CAD build for the part. Positions are in the model's coordinates, mm. A direction names the side the tool comes from. Give positions to 0.01 mm unless a question says otherwise; leave off trailing zeros. Write each loop counter-clockwise with the first axis right and the second up, starting at its lowest first coordinate (ties: lowest second). Pieces come first, ordered by that corner, then holes. Notation, with made-up numbers: (43.25, -26) - (99.25, -26) arc R29 ccw to (99.25, 7) - close; hole circle Ø3 at (8.25, -26.5). An arc over 180 degrees is marked (long way). Put each result on its own line as item: value. Start each with the question number.
1. Cut at C-C on z = 9. List the corners of the cut face in (x, y), and give its area (3 significant figures).
2. Drop flat-ended pins along their axis: pin 1 (8 mm diameter, centred on x = 21, z = -0.5, fed in from -Y); pin 2 (1 mm diameter, centred on x = 44.5, y = 4, fed in from -Z); pin 3 (8 mm diameter, centred on x = 57.5, z = 9, fed in from +Y). Give the stop position or say it passes through.
3. Mould opens along X. For faces 6 (the flat face through (68.9, -2, 9)), 7 (the flat face through (34, 5, 0)), 8 (the flat face through (1, -7, 0)) say: +X half, -X half, draft (parallel to the pull), parting line (faces both ways), or undercut.
4. Tool access for faces 1 (the flat face through (1, -2, 9)), 2 (the cylindrical face through (1.91, -5.48, -52.39)), 3 (the flat face through (21, -2, -63)), 4 (the flat face through (68.9, -2, -63)), 5 (the flat face through (11, -1, -60.9)): list every direction of +Z, -Z, +X, -X, +Y, -Y with a clear straight run to the whole face (end or side of a thin tool).
5. Cut at A-A on z = -27.2. List the corners of the cut face in (x, y).
6. Wall check: line 1 (Y direction, x = -0.45, z = -27.2); line 2 (Z direction, x = 63, y = 9.25); line 3 (Z direction, x = 12.5, y = 0.25). Give the ranges that are in metal, low to high.
7. Cut at D-D on x = 27.5. List the corners of the cut face in (y, z), and give its area (3 significant figures).
8. Cut at B-B on y = 8. List the corners of the cut face in (x, z).
from build123d import *

# Parameters (mm, degrees)
SKETCH1_W               = 77.9
SKETCH1_H               = 62.4
SKETCH1_W_2             = 69.9
SKETCH1_H_2             = 54.4
BOSS_EXTRUDE1_DEPTH     = 10
SKETCH2_W               = 77.9
SKETCH2_H               = 62.4
BOSS_EXTRUDE2_DEPTH     = 4
SKETCH7_W               = 73.9
SKETCH7_H               = 58.4
SKETCH7_W_2             = 69.9
SKETCH7_H_2             = 54.4
BOSS_EXTRUDE4_DEPTH     = 1
CUT_EXTRUDE1_REACH      = 99.979
SKETCH3_W               = 13
SKETCH3_H               = 7.25
CUT_EXTRUDE2_REACH      = 99.979
SKETCH4_W               = 10
SKETCH4_H               = 7.25
SKETCH5_R               = 1.36925
CUT_EXTRUDE4_DEPTH      = 25
SKETCH6_R               = 2.5
BOSS_EXTRUDE3_DEPTH     = 3
SKETCH9_W               = 10
SKETCH9_H               = 1
SKETCH9_W_2             = 13
CUT_EXTRUDE5_DEPTH      = 11
SKETCH11_W              = 5
SKETCH11_H              = 5
SKETCH11_R              = 1
BOSS_EXTRUDE5_DEPTH     = 2
BOSS_EXTRUDE6_START     = -2
SKETCH12_W              = 5
SKETCH12_H              = 5
SKETCH12_R              = 1
BOSS_EXTRUDE6_DEPTH     = 2
SKETCH13_W              = 20
SKETCH13_H              = 5
BOSS_EXTRUDE7_DEPTH     = 10
CUT_EXTRUDE6_DEPTH      = 10
MIRROR2_COPY_1_SKETCH_W = 20
MIRROR2_COPY_1_SKETCH_H = 5
MIRROR2_COPY_1_DEPTH    = 10
MIRROR2_COPY_2_DEPTH    = 10


with BuildPart() as part:
    # Sketch1 → Boss-Extrude1 (new body)
    with BuildSketch(Plane(origin=(0, 0, 0), x_dir=(1, 0, 0), z_dir=(0, 1, 0))):
        with Locations((34.95, 27.2)):
            Rectangle(SKETCH1_W, SKETCH1_H)
        with Locations((34.95, 27.2)):
            Rectangle(SKETCH1_W_2, SKETCH1_H_2, mode=Mode.SUBTRACT)
    extrude(amount=BOSS_EXTRUDE1_DEPTH)

    # Sketch2 → Boss-Extrude2 (add)
    with BuildSketch(Plane(origin=(0, 0, 0), x_dir=(1, 0, 0), z_dir=(0, 1, 0))):
        with Locations((34.95, 27.2)):
            Rectangle(SKETCH2_W, SKETCH2_H)
    extrude(amount=-BOSS_EXTRUDE2_DEPTH)

    # Sketch7 → Boss-Extrude4 (add)
    with BuildSketch(Plane(origin=(0, 10, 0), x_dir=(1, 0, 0), z_dir=(0, 1, 0))):
        with Locations((34.95, 27.2)):
            Rectangle(SKETCH7_W, SKETCH7_H)
        with Locations((34.95, 27.2)):
            Rectangle(SKETCH7_W_2, SKETCH7_H_2, mode=Mode.SUBTRACT)
    extrude(amount=BOSS_EXTRUDE4_DEPTH)

    # Sketch3 → Cut-Extrude1 (cut, up to next)
    with BuildSketch(Plane.ZY.offset(4), mode=Mode.PRIVATE) as cut_extrude1_sk1:
        with Locations((-38.4, 6.375)):
            Rectangle(SKETCH3_W, SKETCH3_H)
    cut_extrude1_tool1 = extrude(cut_extrude1_sk1.sketch, amount=-CUT_EXTRUDE1_REACH, mode=Mode.PRIVATE) & part.part
    add(cut_extrude1_tool1.solids().sort_by_distance((-4, 6.375, -38.4))[0], mode=Mode.SUBTRACT)

    # Sketch4 → Cut-Extrude2 (cut, up to next)
    with BuildSketch(Plane.ZY.offset(4), mode=Mode.PRIVATE) as cut_extrude2_sk1:
        with Locations((-8.5, 6.375)):
            Rectangle(SKETCH4_W, SKETCH4_H)
    cut_extrude2_tool1 = extrude(cut_extrude2_sk1.sketch, amount=-CUT_EXTRUDE2_REACH, mode=Mode.PRIVATE) & part.part
    add(cut_extrude2_tool1.solids().sort_by_distance((-4, 6.375, -8.5))[0], mode=Mode.SUBTRACT)

    # Sketch5 → Cut-Extrude4 (cut, symmetric)
    with BuildSketch(Plane(origin=(0, -4, 0), x_dir=(-1, 0, 0), z_dir=(0, -1, 0))):
        with Locations(Location((-65.94475, 7.99125, 0), (0, 0, 270))):
            Circle(SKETCH5_R)
        with Locations(Location((-15.15745, 51.15855, 0), (0, 0, 270))):
            Circle(SKETCH5_R)
        with Locations(Location((-65.94475, 35.91855, 0), (0, 0, 270))):
            Circle(SKETCH5_R)
        with Locations(Location((-14.01445, 3.24145, 0), (0, 0, 270))):
            Circle(SKETCH5_R)
    extrude(amount=CUT_EXTRUDE4_DEPTH, both=True, mode=Mode.SUBTRACT)

    # Sketch6 → Boss-Extrude3 (add)
    with BuildSketch(Plane(origin=(0, -4, 0), x_dir=(-1, 0, 0), z_dir=(0, -1, 0))):
        with Locations(Location((-0.95, -0.3, 0), (0, 0, 270))):
            Circle(SKETCH6_R)
        with Locations(Location((-0.95, 54.7, 0), (0, 0, 270))):
            Circle(SKETCH6_R)
        with Locations(Location((-68.95, 54.7, 0), (0, 0, 270))):
            Circle(SKETCH6_R)
        with Locations(Location((-68.95, -0.3, 0), (0, 0, 270))):
            Circle(SKETCH6_R)
    extrude(amount=BOSS_EXTRUDE3_DEPTH)

    # Sketch9 → Cut-Extrude5 (cut)
    with BuildSketch(Plane.ZY.offset(2)):
        with Locations((-8.5, 10.5)):
            Rectangle(SKETCH9_W, SKETCH9_H)
        with Locations((-38.4, 10.5)):
            Rectangle(SKETCH9_W_2, SKETCH9_H)
    extrude(amount=-CUT_EXTRUDE5_DEPTH, mode=Mode.SUBTRACT)

    # Sketch11 → Boss-Extrude5 (add)
    with BuildSketch(Plane(origin=(71.9, 0, 0), x_dir=(0, 0, -1), z_dir=(1, 0, 0))):
        with Locations((27.2, 12.5)):
            Rectangle(SKETCH11_W, SKETCH11_H)
        with Locations((27.2, 12.5)):
            Circle(SKETCH11_R, mode=Mode.SUBTRACT)
    extrude(amount=-BOSS_EXTRUDE5_DEPTH)

    # Sketch12 → Boss-Extrude6 (add)
    with BuildSketch(Plane.ZY.offset(2).offset(BOSS_EXTRUDE6_START)):
        with Locations((-27.2, 12.5)):
            Rectangle(SKETCH12_W, SKETCH12_H)
        with Locations(Location((-27.2, 12.5, 0), (0, 0, 180))):
            Circle(SKETCH12_R, mode=Mode.SUBTRACT)
    extrude(amount=BOSS_EXTRUDE6_DEPTH)

    # Sketch13 → Boss-Extrude7 (add)
    with BuildSketch(Plane(origin=(0, 0, -58.4), x_dir=(-1, 0, 0), z_dir=(0, 0, -1))):
        with Locations((-58.9, -1.5)):
            Rectangle(SKETCH13_W, SKETCH13_H)
    boss_extrude7 = extrude(amount=BOSS_EXTRUDE7_DEPTH)

    # Sketch14 → Cut-Extrude6 (cut)
    with BuildSketch(Plane(origin=(0, 1, 0), x_dir=(1, 0, 0), z_dir=(0, 1, 0))):
        with BuildLine():
            Line((63.9, 60.9), (53.9, 60.9))
            ThreePointArc((53.9, 60.9), (51.4, 63.4), (53.9, 65.9))
            Line((53.9, 65.9), (63.9, 65.9))
            ThreePointArc((63.9, 65.9), (66.4, 63.4), (63.9, 60.9))
        make_face()
    cut_extrude6 = extrude(amount=-CUT_EXTRUDE6_DEPTH, mode=Mode.SUBTRACT)

    # Mirror1: Boss-Extrude7, Cut-Extrude6 across plane
    add(boss_extrude7.mirror(Plane(origin=(0, 0, -27.2), x_dir=(1, 0, 0), z_dir=(0, 0, -1))))
    add(cut_extrude6.mirror(Plane(origin=(0, 0, -27.2), x_dir=(1, 0, 0), z_dir=(0, 0, -1))), mode=Mode.SUBTRACT)

    # Mirror2: Boss-Extrude7, Cut-Extrude6 across plane
    add(boss_extrude7.mirror(Plane.ZY.offset(-34.95)))
    add(cut_extrude6.mirror(Plane.ZY.offset(-34.95)), mode=Mode.SUBTRACT)

    # Mirror2 copy 1 sketch → Mirror2 copy 1 (add)
    with BuildSketch(Plane(origin=(69.9, 0, 4), x_dir=(1, 0, 0), z_dir=(0, 0, 1))):
        with Locations((-58.9, -1.5)):
            Rectangle(MIRROR2_COPY_1_SKETCH_W, MIRROR2_COPY_1_SKETCH_H)
    extrude(amount=MIRROR2_COPY_1_DEPTH)

    # Mirror2 copy 2 sketch → Mirror2 copy 2 (cut)
    with BuildSketch(Plane(origin=(69.9, 1, -54.4), x_dir=(-1, 0, 0), z_dir=(0, 1, 0))):
        with BuildLine():
            Line((63.9, 60.9), (53.9, 60.9))
            ThreePointArc((53.9, 60.9), (51.4, 63.4), (53.9, 65.9))
            Line((53.9, 65.9), (63.9, 65.9))
            ThreePointArc((63.9, 65.9), (66.4, 63.4), (63.9, 60.9))
        make_face()
    extrude(amount=-MIRROR2_COPY_2_DEPTH, mode=Mode.SUBTRACT)


solid = part.part
Report:
1. outline: (1, -4) - (3.5, -4) - (3.5, 1) - (1, 1) - close; (18.5, -4) - (21, -4) - (21, 1) - (18.5, 1) - close; (48.9, -4) - (51.4, -4) - (51.4, 1) - (48.9, 1) - close; (66.4, -4) - (68.9, -4) - (68.9, 1) - (66.4, 1) - close
1. area: 50.0 mm²
2. pin 1: stops at y = -4
2. pin 2: stops at z = -58.4
2. pin 3: stops at y = 1
3. face 6: +X half
3. face 7: undercut
3. face 8: draft
4. face 1: +Z, -X, +Y, -Y
4. face 2: -Y
4. face 3: -Z, +Y, -Y
4. face 4: -Z, +X, +Y, -Y
4. face 5: +Y, -Y
5. outline: (-4, -4) - (73.9, -4) - (73.9, 10) - (71.9, 10) - (71.9, 11.5) - (69.9, 11.5) - (69.9, 0) - (0, 0) - (0, 11.5) - (-2, 11.5) - (-2, 10) - (-4, 10) - close; (-2, 13.5) - (0, 13.5) - (0, 15) - (-2, 15) - close; (69.9, 13.5) - (71.9, 13.5) - (71.9, 15) - (69.9, 15) - close
6. line 1: y = -4 to 11.5, 13.5 to 15
6. line 2: z = -58.4 to -54.4, 0 to 4
6. line 3: z = -68.4 to -65.9, -60.9 to -54.4, 0 to 6.5, 11.5 to 14
7. outline: (-4, -58.4) - (10, -58.4) - (10, -56.4) - (11, -56.4) - (11, -54.4) - (0, -54.4) - (0, 0) - (11, 0) - (11, 2) - (10, 2) - (10, 4) - (-4, 4) - close
7. area: 334 mm²
8. outline: (-4, -58.4) - (73.9, -58.4) - (73.9, 4) - (-4, 4) - (-4, -3.5) - (0, -3.5) - (0, 0) - (69.9, 0) - (69.9, -54.4) - (0, -54.4) - (0, -44.9) - (-4, -44.9) - close; (-4, -31.9) - (0, -31.9) - (0, -13.5) - (-4, -13.5) - close
